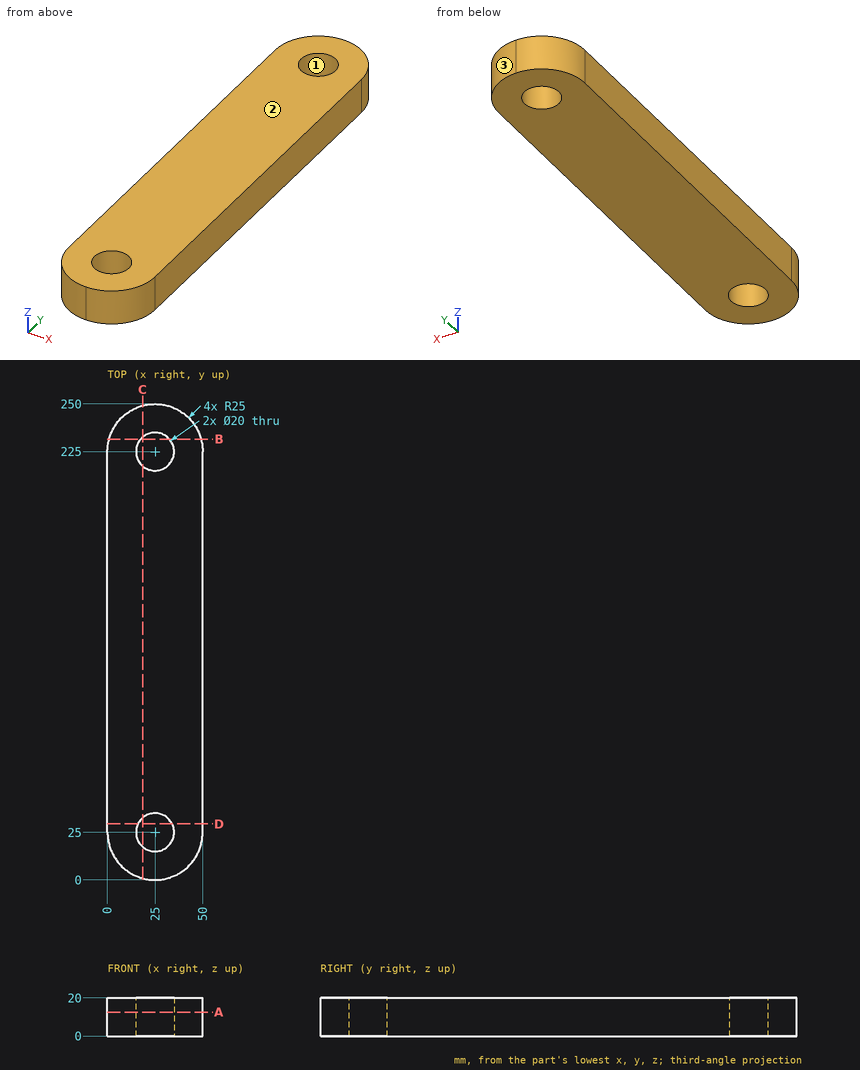
Source: three-view drawing plus pictorial views. Frame: mm from the lowest corner of the part. Give positions to 0.01 mm unless a question says otherwise; leave off trailing zeros. Write each loop counter-clockwise with the first axis right and the second up, starting at its lowest first coordinate (ties: lowest second). Pieces come first, ordered by that corner, then holes. Notation, with made-up numbers: (-10, 88) -> (25, 88) arc R4 cw to (25, 94) -> close; hole circle Ø10 at (1.5, -25). An arc over 180 degrees is marked (long way). Answer in a Markdown table with one row per item.
(1) Section query D-D on y = 29.5. Return loops of the section in (x, z), then the cut area to 3 significant figures.
Answers below:
| item | result |
|---|---|
| outline | (0, 0) -> (16.07, 0) -> (16.07, 20) -> (0, 20) -> close; (33.93, 0) -> (50, 0) -> (50, 20) -> (33.93, 20) -> close |
| area | 643 mm^2 |
(2) Ray query, line 1 along Y through (x, z) = (25, 10.25); line 2 along Y through (x, z) = (26, 11.25); line 3 along X through (y, z) = (26, 17.5). Return the intervals inside material, ascending. Write a range as [from, to].
Answers below:
| item | result |
|---|---|
| line 1 | [0, 15], [35, 215], [235, 250] |
| line 2 | [0.02, 15.05], [34.95, 215.05], [234.95, 249.98] |
| line 3 | [0, 15.05], [34.95, 50] |
(3) Pin query (flat end, axial travel): pin 1 (5 mm diameter, centred on x = 10.5, z = 4.5, fed in from +Y); pin 2 (2 mm diameter, centred on x = 10, z = 6, fed in from -Y). Return the tip coordinate at first contact, or that it passes through.
Answers below:
| item | result |
|---|---|
| pin 1 | y = 246.93 |
| pin 2 | y = 4.29 |
(4) Section query A-A on z = 12.5. State how many separate pieces and enclosed holes the cut face has, then the cut area to 3 significant figures.
Answers below:
| item | result |
|---|---|
| separate pieces | 1 |
| enclosed holes | 2 |
| area | 11,300 mm^2 |
(5) Draft query along Y for the marked faces 1, 2 and 3. Return one class per face: +Y half, -Y half, draft (parallel to the pull), parting line (faces both ways), or undercut.
Answers below:
| item | result |
|---|---|
| face 1 | undercut |
| face 2 | draft |
| face 3 | +Y half |
(6) Section query B-B on y = 231.5. Return loops of the section in (x, z), then the cut area to 3 significant figures.
Answers below:
| item | result |
|---|---|
| outline | (0.86, 0) -> (17.4, 0) -> (17.4, 20) -> (0.86, 20) -> close; (32.6, 0) -> (49.14, 0) -> (49.14, 20) -> (32.6, 20) -> close |
| area | 662 mm^2 |
(7) Section query C-C on x = 18.5. Return loops of the section in (y, z).
Answers below:
| item | result |
|---|---|
| outline | (0.86, 0) -> (17.4, 0) -> (17.4, 20) -> (0.86, 20) -> close; (32.6, 0) -> (217.4, 0) -> (217.4, 20) -> (32.6, 20) -> close; (232.6, 0) -> (249.14, 0) -> (249.14, 20) -> (232.6, 20) -> close |
